Verification items for this drawing (mm, ordinates from the low corner). Coordinates: 2 decimals unless noted, no trailing zeros. Order: outer loops, then holes, each group sorted by start corner. A loop starts at its lowest first (then second) coordinate and runs counter-clockwise, first axis right, second up.
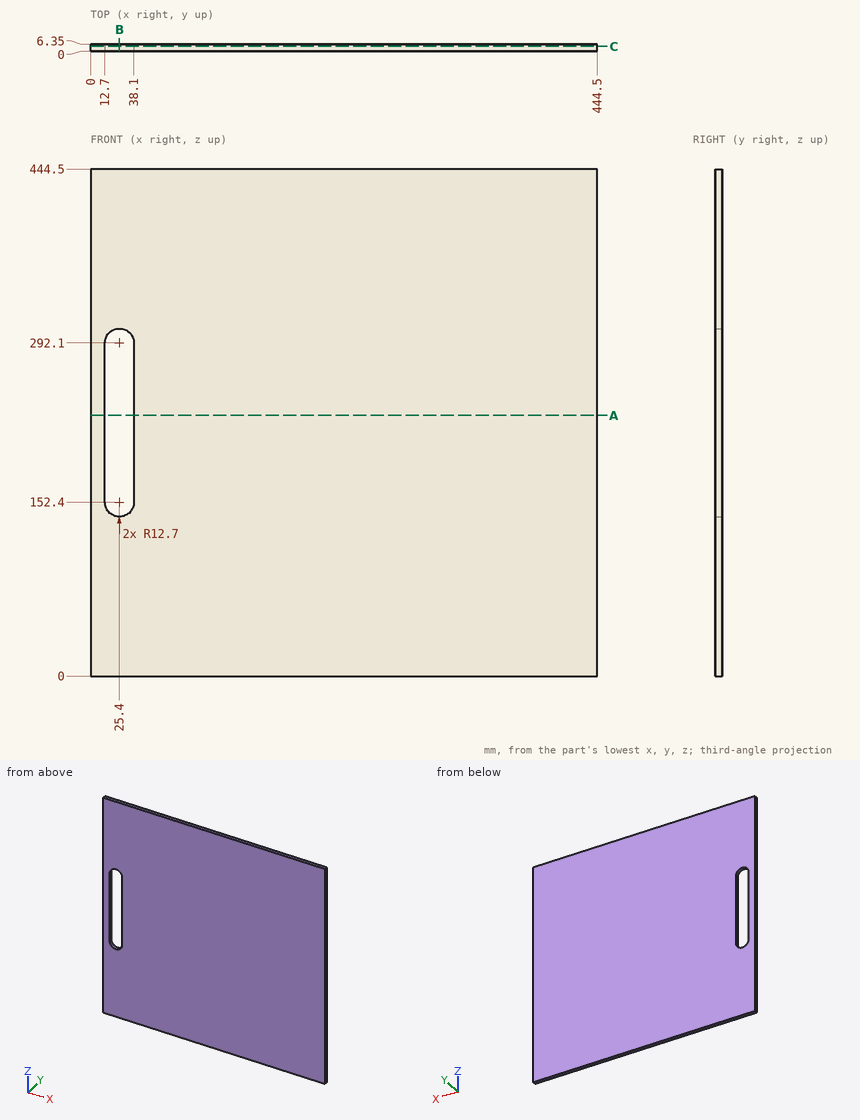
(1) Cross-section at A-A (z = 228.5). Enter the section's corners in (x, y).
Filled in:
outline: (0, 0) - (12.7, 0) - (12.7, 6.35) - (0, 6.35) - close; (38.1, 0) - (444.5, 0) - (444.5, 6.35) - (38.1, 6.35) - close
(2) Thickness scan on probe 1 along X at (y, z) = (2.75, 225); probe 2 along Z at (x, y) = (29.5, 3). Record the ranges inside material, lowest first.
Filled in:
probe 1: x = 0 to 12.7, 38.1 to 444.5
probe 2: z = 0 to 140.38, 304.12 to 444.5
(3) Cross-section at B-B (x = 25.4). Enter the section's corners in (y, z).
Filled in:
outline: (0, 0) - (6.35, 0) - (6.35, 139.7) - (0, 139.7) - close; (0, 304.8) - (6.35, 304.8) - (6.35, 444.5) - (0, 444.5) - close
(4) Cross-section at C-C (y = 4.25). Enter the section's corners in (x, z).
Filled in:
outline: (0, 0) - (444.5, 0) - (444.5, 444.5) - (0, 444.5) - close; hole (12.7, 152.4) arc R12.7 ccw to (38.1, 152.4) - (38.1, 292.1) arc R12.7 ccw to (12.7, 292.1) - close
